from build123d import *

# Parameters (mm, degrees)
SKETCH1_W                           = 14.2875
SKETCH1_H                           = 6.35
EXTRUDE1_DEPTH                      = 44.45
SKETCH6_R                           = 6.3627
CUT_EXTRUDE2_DEPTH                  = 1.27
F_6_32_TAPPED_HOLE1_D               = 2.7051
F_6_32_TAPPED_HOLE1_DEPTH           = 9.398
F_6_32_TAPPED_HOLE1_TIP             = 0.81269403
F_6_32_TAPPED_HOLE1_ON_FACE_2_D     = 2.7051
F_6_32_TAPPED_HOLE1_ON_FACE_2_DEPTH = 9.398
F_6_32_TAPPED_HOLE1_ON_FACE_2_TIP   = 0.81269403


with BuildPart() as part:
    # Sketch1 → Extrude1 (new body)
    with BuildSketch(Plane(origin=(0, 0, 0), x_dir=(1, 0, 0), z_dir=(0, 1, 0))):
        with Locations((-45.973078165, 33.616731266)):
            Rectangle(SKETCH1_W, SKETCH1_H)
    extrude(amount=EXTRUDE1_DEPTH)

    # Sketch6 → Cut-Extrude2 (cut)
    with BuildSketch(Plane.XY.offset(-30.441731266)):
        with Locations((-45.973078165, 30.099)):
            Circle(SKETCH6_R)
    extrude(amount=-CUT_EXTRUDE2_DEPTH, mode=Mode.SUBTRACT)

    # #6-32 Tapped Hole1
    with Locations(Plane(origin=(-45.973078165, 44.45, -33.616731266), x_dir=(0, 0, 1), z_dir=(0, 1, 0))):
        with Locations((0, 0)):
            Hole(F_6_32_TAPPED_HOLE1_D / 2, depth=F_6_32_TAPPED_HOLE1_DEPTH)
            with Locations((0, 0, -(F_6_32_TAPPED_HOLE1_DEPTH + F_6_32_TAPPED_HOLE1_TIP / 2))):  # 118° drill point
                Cone(0, F_6_32_TAPPED_HOLE1_D / 2, F_6_32_TAPPED_HOLE1_TIP, mode=Mode.SUBTRACT)

    # #6-32 Tapped Hole1 on face 2
    with Locations(Plane(origin=(-45.973078165, 0, -33.616731266), x_dir=(0, 0, -1), z_dir=(0, -1, 0))):
        with Locations((0, 0)):
            Hole(F_6_32_TAPPED_HOLE1_ON_FACE_2_D / 2, depth=F_6_32_TAPPED_HOLE1_ON_FACE_2_DEPTH)
            with Locations((0, 0, -(F_6_32_TAPPED_HOLE1_ON_FACE_2_DEPTH + F_6_32_TAPPED_HOLE1_ON_FACE_2_TIP / 2))):  # 118° drill point
                Cone(0, F_6_32_TAPPED_HOLE1_ON_FACE_2_D / 2, F_6_32_TAPPED_HOLE1_ON_FACE_2_TIP, mode=Mode.SUBTRACT)


solid = part.part
The model under review builds one solid part; all positions refer to its coordinate system, in mm. A direction names the side the tool comes from. Coordinates: 2 decimals unless noted, no trailing zeros. Loops run counter-clockwise (first coordinate to the right, second up) from the corner with the lowest first, then second, coordinate; pieces in that order, holes last. Notation, with made-up numbers: M 7,12.25 L 19,12.25 A15 cw 19,33.25 Z; hole C -39,54 d10. An arc over 180 degrees is marked long. Put each result on its own line as item: value. Start each with the question number.
Q1. Add section A-A (x = -43.5). Write out the cut boundary in (y, z).
Q2. The part is to be moulded in two halves that separate along Y. For faces 6 (the flat face through (-46, 44.45, -32)), 7 (the flat face through (-46, 30, -31.712)), 8 (the flat face through (-46, 22, -30.442)), say which applies: +Y half, -Y half, draft (parallel to the pull), parting line (faces both ways), or undercut.
Q3. Add section D-D (y = 41). Write out the cut boundary in (x, z), and give its area (3 significant figures).
Q4. Wall thickness on line 1 (Z direction, x = -40.5, y = 29); line 2 (Y direction, x = -49, z = -31.5); line 3 (X direction, y = 35.5, z = -34.75): over which ranges is each line inside the solid? List them lowest first.
Q5. Add section C-C (y = 25.5). Write out the cut boundary in (x, z).
Q6. Clearance check with a flat-ended pin moving along its axis: pin 1 (2.5 mm diameter, centred on x = -45.97, z = -33.62, fed in from +Y). State where the tip first meets the part, or that it passes through.
Q7. For faces 1 (the cylindrical face through (-52.33, 30.38, -31.07)), 2 (the cylindrical face through (-46.491, 4.765, -32.367)), 3 (the flat face through (-53.117, 22, -34)), 4 (the cylindrical face through (-46.491, 39.685, -34.866)), 5 (the flat face through (-38.829, 22, -34)), list the 3-axis set-ups (+Z, -Z, +X, -X, +Y, -Y) from which the entire face can be reached by the end or side of a thin tool; tool diameter is ignored.
Q8. Add section B-B (z = -31). Write out the cut boundary in (x, y).
Answers:
1. outline: M 0,-36.79 L 44.45,-36.79 L 44.45,-30.44 L 35.96,-30.44 L 35.96,-31.71 L 24.24,-31.71 L 24.24,-30.44 L 0,-30.44 Z
2. face 6: +Y half
2. face 7: undercut
2. face 8: draft
3. outline: M -53.12,-36.79 L -38.83,-36.79 L -38.83,-30.44 L -53.12,-30.44 Z; hole C -45.97,-33.62 d2.71
3. area: 85.0 mm^2
4. line 1: z = -36.79 to -31.71
4. line 2: y = 0 to 24.5, 35.7 to 44.45
4. line 3: x = -53.12 to -46.71, -45.23 to -38.83
5. outline: M -53.12,-36.79 L -38.83,-36.79 L -38.83,-30.44 L -41.58,-30.44 L -41.58,-31.71 L -50.37,-31.71 L -50.37,-30.44 L -53.12,-30.44 Z
6. pin 1: stops at y = 34.99
7. face 1: +Z
7. face 2: -Y
7. face 3: +Z, -Z, -X, +Y, -Y
7. face 4: +Y
7. face 5: +Z, -Z, +X, +Y, -Y
8. outline: M -53.12,0 L -38.83,0 L -38.83,44.45 L -53.12,44.45 Z; hole C -45.97,30.1 d12.73
